Read the model definition and answer for the solid it produces. Units are mm, in the model's axes. Give positions to 0.01 mm unless a question says otherwise; leave off trailing zeros. Write each loop counter-clockwise with the first axis right and the second up, starting at its lowest first coordinate (ties: lowest second). Pieces come first, ordered by that corner, then holes.
```python
from build123d import *

# Parameters (mm, degrees)
F0_W     = 200
F0_H     = 90
F1_DEPTH = 20
F2_R     = 2.5
F3_DEPTH = 15


with BuildPart() as f1:
    # F0 (on Top) → F1 (new body)
    with BuildSketch(Plane.XY):
        Rectangle(F0_W, F0_H)
    extrude(amount=F1_DEPTH)

    # F2 (on face) → F3 (join)
    with BuildSketch(Plane.XY.offset(20)):
        with Locations((-60, 0)):
            Circle(F2_R)
        with Locations((-42, 0)):
            Circle(F2_R)
        with Locations((-22, 0)):
            Circle(F2_R)
        Circle(F2_R)
        with Locations((24, 0)):
            Circle(F2_R)
        with Locations((50, 0)):
            Circle(F2_R)
    extrude(amount=F3_DEPTH)


solid = f1.part
```
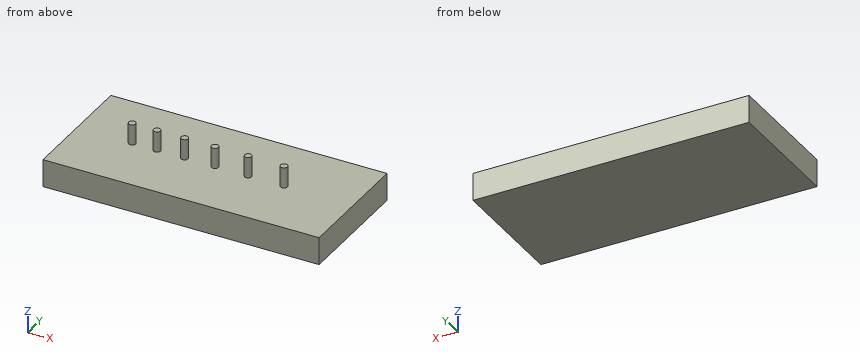
Item 1: Section A-A (z = 29) is taken. Write down the section's boundary in (x, y), and give its area (3 significant figures).
Result set:
outline: circle Ø5 at (-60, 0); circle Ø5 at (-42, 0); circle Ø5 at (-22, 0); circle Ø5 at (0, 0); circle Ø5 at (24, 0); circle Ø5 at (50, 0)
area: 118 mm2
Item 2: Section D-D (y = -18.5) is taken. Write down the section's boundary in (x, z), and give its area (3 significant figures).
Result set:
outline: (-100, 0) - (100, 0) - (100, 20) - (-100, 20) - close
area: 4,000 mm2
Item 3: This flat-tipped pin is pushed along its axis until it touches: pin 1 Ø2 at (x, y) = (-30.5, 20.5) entering from +Z. Where does it stop, or does it pass through?
Result set:
pin 1: stops at z = 20
Item 4: Section C-C (x = 0) is taken. Write down the section's boundary in (y, z), and give its area (4 significant figures).
Result set:
outline: (-45, 0) - (45, 0) - (45, 20) - (2.5, 20) - (2.5, 35) - (-2.5, 35) - (-2.5, 20) - (-45, 20) - close
area: 1,875 mm2
Item 5: Section B-B (y = 0) is taken. Write down the section's boundary in (x, z), and give its area (3 significant figures).
Result set:
outline: (-100, 0) - (100, 0) - (100, 20) - (52.5, 20) - (52.5, 35) - (47.5, 35) - (47.5, 20) - (26.5, 20) - (26.5, 35) - (21.5, 35) - (21.5, 20) - (2.5, 20) - (2.5, 35) - (-2.5, 35) - (-2.5, 20) - (-19.5, 20) - (-19.5, 35) - (-24.5, 35) - (-24.5, 20) - (-39.5, 20) - (-39.5, 35) - (-44.5, 35) - (-44.5, 20) - (-57.5, 20) - (-57.5, 35) - (-62.5, 35) - (-62.5, 20) - (-100, 20) - close
area: 4,450 mm2
Item 6: Find the intervals of material crossed by line 1 along Z through (x, y) = (59, -33); line 2 along Y through (x, z) = (-61, 21); line 3 along Y through (x, z) = (-40, 23.5), in increasing order.
Result set:
line 1: z = 0 to 20
line 2: y = -2.29 to 2.29
line 3: y = -1.5 to 1.5
